Geometry: final body of the model. Coordinates: model frame, mm. A direction names the side the tool comes from. Give positions to 0.01 mm unless a question says otherwise; leave off trailing zeros. Write each loop counter-clockwise with the first axis right and the second up, starting at its lowest first coordinate (ties: lowest second). Pieces come first, ordered by that corner, then holes. Notation, with made-up numbers: M 10,-9 L 32,-9 A35 ccw 32,25 Z; hole C 86.5,85.25 d1. An arc over 180 degrees is marked long. One line per question, with ' | ' between items.
from build123d import *
from build123d import SkipClean  # not in build123d's __all__

# Parameters (mm, degrees)
F1_DEPTH    = 10
F3_DEPTH    = 4
F5_DEPTH    = 4
F6_R        = 0.5
F7_T1_DEPTH = 20
F7_T3_DEPTH = 4.5763046334


# Not quite as in the source:
# - a fillet or chamfer that OpenCascade refuses, or shapes differently, is made with other operations: its cross-section is extruded or revolved along the edge and cut away or added


with BuildPart() as f1:
    # F0 (on Front) → F1 (new body, symmetric)
    with BuildSketch(Plane.XZ):
        with BuildLine():
            Line((-2.4494897428, 0), (2.4494897428, 0))
            ThreePointArc((2.4494897428, 0), (0, 6), (-2.4494897428, 0))
        make_face()
    extrude(amount=F1_DEPTH, both=True)

    # F2 (on face) → F3 (join)
    with BuildSketch(Plane.XZ.offset(10)):
        with BuildLine():
            Line((-2.4494897428, 5), (-7, 5))
            Line((-7, 5), (-7, 0))
            Line((-7, 0), (-2.4494897428, 0))
            ThreePointArc((-2.4494897428, 0), (-3.5, 2.5), (-2.4494897428, 5))
        make_face()
        with BuildLine():
            Line((2.4494897428, 5), (-2.4494897428, 5))
            ThreePointArc((-2.4494897428, 5), (-3.5, 2.5), (-2.4494897428, 0))
            Line((-2.4494897428, 0), (2.4494897428, 0))
            ThreePointArc((2.4494897428, 0), (3.5, 2.5), (2.4494897428, 5))
        make_face()
        with BuildLine():
            Line((7, 5), (2.4494897428, 5))
            ThreePointArc((2.4494897428, 5), (3.5, 2.5), (2.4494897428, 0))
            Line((2.4494897428, 0), (7, 0))
            Line((7, 0), (7, 5))
        make_face()
    extrude(amount=F3_DEPTH)

    # F4 (on face) → F5 (join)
    with BuildSketch(Plane(origin=(0, 10, 0), x_dir=(-1, 0, 0), z_dir=(0, 1, 0))):
        with BuildLine():
            ThreePointArc((-2.4494897428, 5), (-3.5, 2.5), (-2.4494897428, 0))
            Line((-2.4494897428, 0), (2.4494897428, 0))
            ThreePointArc((2.4494897428, 0), (3.5, 2.5), (2.4494897428, 5))
            Line((2.4494897428, 5), (-2.4494897428, 5))
        make_face()
    extrude(amount=F5_DEPTH)

    # F6
    f6_edges = [f1.edges().sort_by_distance(p)[0] for p in [
        (7, -12, 5),
        (7, -12, 0),
        (-7, -12, 5),
        (-7, -12, 0),
    ]]
    fillet(f6_edges, radius=F6_R)

    # F7: fillet of radius 0.5 on 6 edges, made by hand

    # F7_s2 → F7_t1 (cut)
    with BuildSketch(Plane.XZ.offset(-10)):
        with BuildLine():
            ThreePointArc((2.2360679775, 0), (2.4401921227, 0.0435645354), (2.6087459737, 0.1666666667))
            ThreePointArc((2.6087459737, 0.1666666667), (2.5304903844, 0.0820218333), (2.4494897428, 0))
            Line((2.4494897428, 0), (2.2360679775, 0))
        make_face()
        with BuildLine():
            ThreePointArc((-2.2360679775, 0), (-2.4401921227, 0.0435645354), (-2.6087459737, 0.1666666667))
            ThreePointArc((-2.6087459737, 0.1666666667), (-2.5304903844, 0.0820218333), (-2.4494897428, 0))
            Line((-2.4494897428, 0), (-2.2360679775, 0))
        make_face()
    with SkipClean():  # cleaning this boolean's faces spoils the solid; the shape is the same uncleaned
        extrude(amount=F7_T1_DEPTH, mode=Mode.SUBTRACT)

    # F7_s4 → F7_t3 (cut)
    with BuildSketch(Plane.XZ.offset(-14.5763046334)):
        with BuildLine():
            ThreePointArc((2.2360679775, 0), (2.4401921227, 0.0435645354), (2.6087459737, 0.1666666667))
            ThreePointArc((2.6087459737, 0.1666666667), (2.5304903844, 0.0820218333), (2.4494897428, 0))
            Line((2.4494897428, 0), (2.2360679775, 0))
        make_face()
        with BuildLine():
            ThreePointArc((-2.2360679775, 0), (-2.4401921227, 0.0435645354), (-2.6087459737, 0.1666666667))
            ThreePointArc((-2.6087459737, 0.1666666667), (-2.5304903844, 0.0820218333), (-2.4494897428, 0))
            Line((-2.4494897428, 0), (-2.2360679775, 0))
        make_face()
        with BuildLine():
            ThreePointArc((2.6087459737, 4.8333333333), (2.4401921227, 4.9564354646), (2.2360679775, 5))
            Line((2.2360679775, 5), (2.4494897428, 5))
            ThreePointArc((2.4494897428, 5), (2.5304903844, 4.9179781667), (2.6087459737, 4.8333333333))
        make_face()
        with BuildLine():
            ThreePointArc((-2.6087459737, 4.8333333333), (-2.4401921227, 4.9564354646), (-2.2360679775, 5))
            Line((-2.2360679775, 5), (-2.4494897428, 5))
            ThreePointArc((-2.4494897428, 5), (-2.5304903844, 4.9179781667), (-2.6087459737, 4.8333333333))
        make_face()
    extrude(amount=F7_T3_DEPTH, mode=Mode.SUBTRACT)


solid = f1.part
(1) Cut plane C-C, the plane y = -6.5. Return loops of the section in (x, z), then the cut area to 3 significant figures.
Working result:
outline: M -2.61,0.17 A0.5 ccw -2.24,0 L 2.24,0 A0.5 ccw 2.61,0.17 A3.5 ccw long Z | area: 35.1 mm^2
(2) Cut plane A-A, the plane y = 12.25. Return loops of the section in (x, z), then the cut area to 3 significant figures.
Working result:
outline: M -2.61,0.17 A0.5 ccw -2.24,0 L 2.24,0 A0.5 ccw 2.61,0.17 A3.5 ccw 2.61,4.83 A0.5 ccw 2.24,5 L -2.24,5 A0.5 ccw -2.61,4.83 A3.5 ccw Z | area: 31.7 mm^2
(3) Cut plane D-D, the plane z = 5.5. Return loops of the section in (x, y), then the cut area to 3 significant figures.
Working result:
outline: M -1.8,-10 L 1.8,-10 L 1.8,10 L -1.8,10 Z | area: 72.1 mm^2
(4) Cut plane B-B, the plane z = 2.5. Return loops of the section in (x, y).
Working result:
outline: M -7,-14 L 7,-14 L 7,-10 L 3.5,-10 L 3.5,14 L -3.5,14 L -3.5,-10 L -7,-10 Z
(5) Material intervals for L1, parallel to Y at x = 6.5, z = 1.7; L2, parallel to X at y = 2, z = 2.35; L3, parallel to Z at x = 3.75, y = -12, sorted ascending. Write a range as [from, to].
Working result:
L1: y = [-14, -10] | L2: x = [-3.5, 3.5] | L3: z = [0, 5]
(6) First-contact query: P1, Ø3, axis at x = 1, y = 12, coming from the +Z side; P2, Ø1.5, axis at y = 8.5, z = 2.5, coming from the -X side; P3, Ø2, axis at x = -3.5, y = 7, coming from the +Z side. Flat tips, straight axial feed; report the tip coordinate or a pass-through.
Working result:
P1: stops at z = 5 | P2: stops at x = -3.5 | P3: stops at z = 4.95
(7) Draft query along X for faces 4 (the face through (7, -12, 2)), 5 (the face through (0, -10, 5.4)), 6 (the face through (-7, -12, 3)). Return one class per face: released by +X, released by -X, zero draft, split by the parting line, or undercut.
Working result:
face 4: released by +X | face 5: zero draft | face 6: released by -X
(8) Set-up query: faces 1 (the face through (0, -12, 5)), 2 (the face through (0, -14, 3)), 3 (the face through (0, 12, 5)). Return all of +Z, -Z, +X, -X, +Y, -Y with unobstructed straight access to the full face (end or side cutting, diameter ignored); none if empty.
Working result:
face 1: +Z, +X, -X, -Y | face 2: +Z, -Z, +X, -X, -Y | face 3: +Z, +X, -X, +Y
